Input: part model. Units: mm. Frame: model coordinates. Face numbers are marked on the shaded views. Round coordinates to 2 decimals unless told otherwise and drop trailing zeros. Write each loop counter-clockwise with the first axis right and the second up, starting at its lowest first coordinate (ties: lowest second). Pieces come first, ordered by that corner, then holes. Notation, with made-up numbers: M -6.75,-18 L 16.25,-18 A16 ccw 16.25,-3 Z; hole C 30.5,78.25 d2. An arc over 180 degrees is marked long. Write each question's results on one line, items separated by ' | '. Start each with the question number.
```python
from build123d import *

# Parameters (mm, degrees)
SKETCH1_W           = 47.5
SKETCH1_H           = 65
BOSS_EXTRUDE1_DEPTH = 22
SKETCH2_R           = 1.6
CUT_EXTRUDE1_DEPTH  = 46.87278605
SKETCH4_W           = 20
SKETCH4_H           = 5
CUT_EXTRUDE2_DEPTH  = 15


with BuildPart() as part:
    # Sketch1 → Boss-Extrude1 (new body)
    with BuildSketch(Plane(origin=(0, 0, 0), x_dir=(1, 0, 0), z_dir=(0, 1, 0))):
        Rectangle(SKETCH1_W, SKETCH1_H)
    extrude(amount=BOSS_EXTRUDE1_DEPTH)

    # Sketch2 → Cut-Extrude1 (cut, through all)
    with BuildSketch(Plane(origin=(0, 22, 0), x_dir=(1, 0, 0), z_dir=(0, 1, 0))):
        with Locations(Location((-13.26, 29.225, 0), (0, 0, 270))):
            Circle(SKETCH2_R)
        with Locations(Location((13.26, 29.225, 0), (0, 0, 270))):
            Circle(SKETCH2_R)
        with Locations(Location((13.26, -29.225, 0), (0, 0, 270))):
            Circle(SKETCH2_R)
        with Locations(Location((-13.26, -29.225, 0), (0, 0, 270))):
            Circle(SKETCH2_R)
    extrude(amount=-CUT_EXTRUDE1_DEPTH, mode=Mode.SUBTRACT)

    # Sketch4 → Cut-Extrude2 (cut)
    with BuildSketch(Plane(origin=(0, 22, 0), x_dir=(1, 0, 0), z_dir=(0, 1, 0))):
        with Locations((0, -30)):
            Rectangle(SKETCH4_W, SKETCH4_H)
    extrude(amount=-CUT_EXTRUDE2_DEPTH, mode=Mode.SUBTRACT)


solid = part.part
```
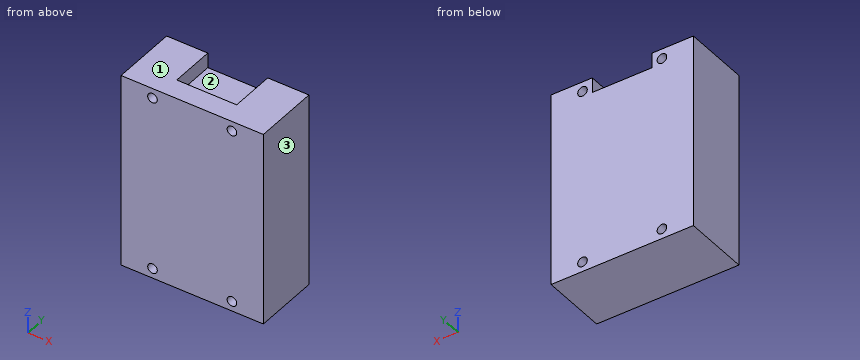
1. Draft query along X for the marked faces 1, 2 and 3. Return one class per face: +X half, -X half, draft (parallel to the pull), parting line (faces both ways), or undercut.
2. Cut plane C-C on x = -1. Output: boundary loops of the cut face in (y, z).
3. Line query: L1, parallel to Z at x = -14.5, y = 8.75; L2, parallel to Z at x = -4.5, y = 10.5; L3, parallel to Y at x = 0.5, z = 29. Output: solid intervals per line, ascending. Write a range as from..to.
4. Contact query for a flat-ended pin moving along its axis: P1, Ø7.5, axis at x = -2, y = 14.5, coming from the +Z side. Output: stop coordinate, or through.
5. Cut plane A-A on y = 18. Output: boundary loops of the cut face in (x, z) (3 decimals).
6. Cut plane B-B on x = 13.26. Output: boundary loops of the cut face in (y, z) (3 decimals).
Answers follow:
1) face 1: draft | face 2: undercut | face 3: +X half
2) outline: M 0,-32.5 L 22,-32.5 L 22,27.5 L 7,27.5 L 7,32.5 L 0,32.5 Z
3) L1: z = -32.5..-30.24, -28.21..28.21, 30.24..32.5 | L2: z = -32.5..27.5 | L3: y = 0..7
4) P1: stops at z = 27.5
5) outline: M -23.75,-32.5 L 23.75,-32.5 L 23.75,32.5 L 10,32.5 L 10,27.5 L -10,27.5 L -10,32.5 L -23.75,32.5 Z; hole C -13.26,-29.225 d3.2; hole C -13.26,29.225 d3.2; hole C 13.26,-29.225 d3.2; hole C 13.26,29.225 d3.2
6) outline: M 0,-32.5 L 22,-32.5 L 22,-30.825 L 0,-30.825 Z; M 0,-27.625 L 22,-27.625 L 22,27.625 L 0,27.625 Z; M 0,30.825 L 22,30.825 L 22,32.5 L 0,32.5 Z
